Here's how the part is built. I have some questions about the finished solid (model axes, mm). A direction names the side the tool comes from. Coordinates: 2 decimals unless noted, no trailing zeros. Loops run counter-clockwise (first coordinate to the right, second up) from the corner with the lowest first, then second, coordinate; pieces in that order, holes last. Notation, with made-up numbers: M 32,57.5 L 81,57.5 A12 ccw 81,63.5 Z; hole C 57,43.25 d7. An arc over 180 degrees is marked long. Use one line per item in the form item = value. Start each with the question number.
(1) Imagine slicing it at D-D, the plane y = -13.5. Please give me the cut outline in (x, z), and give its area (3 significant figures).
(2) Will these pins go through, and if not, where does the flat tip stop? P1, Ø1.5, axis at y = -1, z = 1, coming from the +X side; P2, Ø1, axis at x = 11, z = 2.5, coming from the -Y side; P3, Ø1, axis at x = -17, z = 0.5, coming from the -Y side.
(3) On a 3-axis mill with a long thin cutter (end or side, diameter ignored), from which of +Z, -Z, +X, -X, +Y, -Y can I reach the whole of each face in a straight line? I mean faces 1 (the cylindrical face through (-4.336, -19.524, 2.26)), 2 (the flat face through (-11, 17, 3)). Say none if no direction works.
(4) Please list where these lines run through material, in increasing order: L1, parallel to Y at x = 0, z = 2.5; L2, parallel to Y at x = -3, z = 1.8; L3, parallel to Y at x = 8, z = 1.55.
(5) Thinking about a two-plate mould opening in Y: for faces 3 (the cylindrical face through (-1.08, -4.88, 2.26)), 4 (the flat face through (10, -3, 3)), 5 (the cylindrical face through (23.846, 7.509, 1.479)), which applies, +Y half, -Y half, draft (parallel to the pull), parting line (faces both ways), or undercut?
(6) Imagine slicing it at A-A, the plane y = 0. Please give me the cut outline in (x, z), and give its area (3 significant figures).
(7) Imagine slicing it at C-C, the plane z = 0.75. Please give me the cut outline in (x, y).
```python
from build123d import *

# Parameters (mm, degrees)
F0_R     = 25
F1_DEPTH = 3
F2_R     = 20
F2_R_2   = 15
F2_R_3   = 10
F2_R_4   = 5
F3_DEPTH = 1.5


with BuildPart() as f1:
    # F0 (on Top) → F1 (new body)
    with BuildSketch(Plane.XY):
        Circle(F0_R)
    extrude(amount=F1_DEPTH)

    # F2 (on face) → F3 (cut)
    with BuildSketch(Plane.XY.offset(3)):
        Circle(F2_R)
        Circle(F2_R_2, mode=Mode.SUBTRACT)
        Circle(F2_R_3)
        Circle(F2_R_4, mode=Mode.SUBTRACT)
    extrude(amount=-F3_DEPTH, mode=Mode.SUBTRACT)


solid = f1.part
```
Answer:
q1.outline = M -21.04,0 L 21.04,0 L 21.04,3 L 14.76,3 L 14.76,1.5 L 6.54,1.5 L 6.54,3 L -6.54,3 L -6.54,1.5 L -14.76,1.5 L -14.76,3 L -21.04,3 Z
q1.area = 102 mm²
q2.P1 = 25
q2.P2 = -22.69
q2.P3 = -18.78
q3.face_1 = +Z
q3.face_2 = +Z, +X, -X, +Y, -Y
q4.L1 = -25 to -20, -15 to -10, -5 to 5, 10 to 15, 20 to 25
q4.L2 = -24.82 to -19.77, -14.7 to -9.54, -4 to 4, 9.54 to 14.7, 19.77 to 24.82
q4.L3 = -23.69 to -18.33, -12.69 to -6, 6 to 12.69, 18.33 to 23.69
q5.face_3 = undercut
q5.face_4 = draft
q5.face_5 = parting line
q6.outline = M -25,0 L 25,0 L 25,3 L 20,3 L 20,1.5 L 15,1.5 L 15,3 L 10,3 L 10,1.5 L 5,1.5 L 5,3 L -5,3 L -5,1.5 L -10,1.5 L -10,3 L -15,3 L -15,1.5 L -20,1.5 L -20,3 L -25,3 Z
q6.area = 120 mm²
q7.outline = C 0,0 d50
